```python
from build123d import *

# Parameters (mm, degrees)
F0_W          = 111
F0_H          = 107
F0_W_2        = 13
F0_H_2        = 5
F0_W_3        = 39
F0_H_3        = 7
F0_W_4        = 12
F0_H_4        = 1.5
F0_R          = 2.75
F0_W_5        = 4.5
F0_H_5        = 10
F0_H_6        = 15
F0_W_6        = 14
F0_W_7        = 17
F1_DEPTH      = 23
F2_W          = 111
F2_H          = 107
F3_DEPTH      = 3
F4_DEPTH      = 5
F5_DEPTH      = 13
F7_DEPTH      = 50
F9_DEPTH      = 10
F10_R         = 5
F11_T3_ANGLE  = 90
F11_T6_ANGLE  = 90
F11_T9_ANGLE  = 90
F11_T12_ANGLE = 90
F11_T15_DEPTH = 48
F11_T18_DEPTH = 48
F11_T21_DEPTH = 48
F11_T24_DEPTH = 48
F12_R         = 1


# Not quite as in the source:
# - a fillet or chamfer that OpenCascade refuses, or shapes differently, is made with other operations: its cross-section is extruded or revolved along the edge and cut away or added


with BuildPart() as f1:
    # F0 (on Top) → F1 (new body)
    with BuildSketch(Plane.XY):
        with Locations((55.5, 53.5)):
            Rectangle(F0_W, F0_H)
        with Locations((16.5, 12.5)):
            Rectangle(F0_W_2, F0_H_2, mode=Mode.SUBTRACT)
        Polygon((35.5980762114, 15), (36.4641016151, 13.5), (35.5980762114, 12), (33.8660254038, 12), (33, 13.5), (33.8660254038, 15), align=None, mode=Mode.SUBTRACT)
        with Locations((29.5, 28.5)):
            Rectangle(F0_W_3, F0_H_3, mode=Mode.SUBTRACT)
        with Locations((62.4641016151, 14.25)):
            Rectangle(F0_W_4, F0_H_4, mode=Mode.SUBTRACT)
        with Locations((71.75, 39.25)):
            Circle(F0_R, mode=Mode.SUBTRACT)
        with Locations((91.75, 37)):
            Rectangle(F0_W_5, F0_H_5, mode=Mode.SUBTRACT)
        with Locations((16.5, 59.5)):
            Rectangle(F0_W_2, F0_H_6, mode=Mode.SUBTRACT)
        with Locations((17, 89.5)):
            Rectangle(F0_W_6, F0_H_6, mode=Mode.SUBTRACT)
        with Locations((94.5, 59.5)):
            Rectangle(F0_W_2, F0_H_6, mode=Mode.SUBTRACT)
        with Locations((92.5, 93.5)):
            Rectangle(F0_W_7, F0_H_3, mode=Mode.SUBTRACT)
    extrude(amount=F1_DEPTH)

    # F2 (on face) → F3 (join)
    with BuildSketch(Plane(origin=(0, 0, 0), x_dir=(1, 0, 0), z_dir=(0, 0, -1))):
        with Locations((55.5, -53.5)):
            Rectangle(F2_W, F2_H)
    extrude(amount=-F3_DEPTH)

    # F4 (add): a face of the model
    f4_faces = [f1.faces().sort_by_distance(p)[0] for p in [
        (16.5, 12.5, 3),
    ]]
    extrude(f4_faces, amount=F4_DEPTH)

    # F5 (add): a face of the model
    f5_faces = [f1.faces().sort_by_distance(p)[0] for p in [
        (62.4641016151, 14.25, 3),
    ]]
    extrude(f5_faces, amount=F5_DEPTH)

    # F6 (on face) → F7 (join)
    with BuildSketch(Plane.YZ.offset(111)):
        with BuildLine():
            Line((11.0735931288, 23), (0, 23))
            Line((0, 23), (0, 0))
            Line((0, 0), (107, 0))
            Line((107, 0), (107, 23))
            Line((107, 23), (95.9264068712, 23))
            ThreePointArc((95.9264068712, 23), (53.5, 3), (11.0735931288, 23))
        make_face()
    extrude(amount=F7_DEPTH)

    # F8 (on face) → F9 (join)
    with BuildSketch(Plane.YZ.offset(161)):
        with BuildLine():
            Line((0, 23), (0, 0))
            Line((0, 0), (107, 0))
            Line((107, 0), (107, 23))
            Line((107, 23), (95.9264068712, 23))
            ThreePointArc((95.9264068712, 23), (53.5, 3), (11.0735931288, 23))
            Line((11.0735931288, 23), (0, 23))
        make_face()
        with BuildLine():
            Line((95.9264068712, 23), (11.0735931288, 23))
            ThreePointArc((11.0735931288, 23), (53.5, 3), (95.9264068712, 23))
        make_face()
    extrude(amount=F9_DEPTH)

    # F10
    f10_edges = [f1.edges().sort_by_distance(p)[0] for p in [
        (85.5, 107, 23),
        (171, 53.5, 23),
        (85.5, 0, 23),
        (0, 53.5, 23),
    ]]
    fillet(f10_edges, radius=F10_R)

    # F11: fillet of radius 10 on 4 edges, made by hand


with BuildPart() as f11_tool1:
    # F11_s2 → F11_t3 (revolve)
    with BuildSketch(Plane.YZ.offset(10)):
        with BuildLine():
            ThreePointArc((102, 23), (105.5355339059, 21.5355339059), (107, 18))
            Line((107, 18), (107, 23))
            Line((107, 23), (102, 23))
        make_face()
    revolve(axis=Axis((10, 97, 23), (0, 0, 1)), revolution_arc=F11_T3_ANGLE)


with BuildPart() as f11_tool4:
    # F11_s5 → F11_t6 (revolve)
    with BuildSketch(Plane.XZ.offset(-10)):
        with BuildLine():
            ThreePointArc((5, 23), (1.4644660941, 21.5355339059), (0, 18))
            Line((0, 18), (0, 23))
            Line((0, 23), (5, 23))
        make_face()
    revolve(axis=Axis((10, 10, 23), (0, 0, 1)), revolution_arc=F11_T6_ANGLE)


with BuildPart() as f11_tool7:
    # F11_s8 → F11_t9 (revolve)
    with BuildSketch(Plane.YZ.offset(161)):
        with BuildLine():
            ThreePointArc((5, 23), (1.4644660941, 21.5355339059), (0, 18))
            Line((0, 18), (0, 23))
            Line((0, 23), (5, 23))
        make_face()
    revolve(axis=Axis((161, 10, 23), (0, 0, 1)), revolution_arc=F11_T9_ANGLE)


with BuildPart() as f11_tool10:
    # F11_s11 → F11_t12 (revolve)
    with BuildSketch(Plane.XZ.offset(-97)):
        with BuildLine():
            ThreePointArc((166, 23), (169.5355339059, 21.5355339059), (171, 18))
            Line((171, 18), (171, 23))
            Line((171, 23), (166, 23))
        make_face()
    revolve(axis=Axis((161, 97, 23), (0, 0, 1)), revolution_arc=F11_T12_ANGLE)


with BuildPart() as f11_tool13:
    # F11_s14 → F11_t15 (new body)
    with BuildSketch(Plane.XY.offset(-25)):
        with BuildLine():
            ThreePointArc((161, 107), (168.0710678119, 104.0710678119), (171, 97))
            Line((171, 97), (171, 107))
            Line((171, 107), (161, 107))
        make_face()
    extrude(amount=F11_T15_DEPTH)


with BuildPart() as f11_tool16:
    # F11_s17 → F11_t18 (new body)
    with BuildSketch(Plane.XY.offset(23)):
        with BuildLine():
            ThreePointArc((161, 0), (168.0710678119, 2.9289321881), (171, 10))
            Line((171, 10), (171, 0))
            Line((171, 0), (161, 0))
        make_face()
    extrude(amount=-F11_T18_DEPTH)


with BuildPart() as f11_tool19:
    # F11_s20 → F11_t21 (new body)
    with BuildSketch(Plane.XY.offset(-25)):
        with BuildLine():
            ThreePointArc((0, 10), (2.9289321881, 2.9289321881), (10, 0))
            Line((10, 0), (0, 0))
            Line((0, 0), (0, 10))
        make_face()
    extrude(amount=F11_T21_DEPTH)


with BuildPart() as f11_tool22:
    # F11_s23 → F11_t24 (new body)
    with BuildSketch(Plane.XY.offset(23)):
        with BuildLine():
            ThreePointArc((0, 97), (2.9289321881, 104.0710678119), (10, 107))
            Line((10, 107), (0, 107))
            Line((0, 107), (0, 97))
        make_face()
    extrude(amount=-F11_T24_DEPTH)


with BuildPart() as f1_1:
    add(f1.part)

    # F11_t25: cut F11_tool1, F11_tool4, F11_tool7, F11_tool10, F11_tool13, F11_tool16, F11_tool19, F11_tool22
    add([f11_tool1.part, f11_tool4.part, f11_tool7.part, f11_tool10.part, f11_tool13.part, f11_tool16.part, f11_tool19.part, f11_tool22.part], mode=Mode.SUBTRACT)

    # F12
    f12_edges = [f1_1.edges().sort_by_distance(p)[0] for p in [
        (85.5, 102, 23),
        (164.535534, 100.535534, 23),
        (166, 53.5, 23),
        (164.535534, 6.464466, 23),
        (85.5, 5, 23),
        (6.464466, 6.464466, 23),
        (5, 53.5, 23),
        (6.464466, 100.535534, 23),
        (10, 12.5, 23),
        (16.5, 10, 23),
        (16.5, 15, 23),
        (23, 12.5, 23),
        (36.031089, 14.25, 23),
        (34.732051, 15, 23),
        (36.031089, 12.75, 23),
        (33.433013, 14.25, 23),
        (34.732051, 12, 23),
        (33.433013, 12.75, 23),
        (10, 28.5, 23),
        (29.5, 25, 23),
        (29.5, 32, 23),
        (49, 28.5, 23),
        (56.464102, 14.25, 23),
        (62.464102, 13.5, 23),
        (62.464102, 15, 23),
        (68.464102, 14.25, 23),
        (69, 39.25, 23),
        (89.5, 37, 23),
        (91.75, 32, 23),
        (91.75, 42, 23),
        (94, 37, 23),
        (136, 11.073593, 23),
        (111, 53.5, 23),
        (161, 53.5, 23),
        (136, 95.926407, 23),
        (10, 59.5, 23),
        (16.5, 52, 23),
        (16.5, 67, 23),
        (23, 59.5, 23),
        (17, 82, 23),
        (24, 89.5, 23),
        (10, 89.5, 23),
        (17, 97, 23),
        (94.5, 67, 23),
        (88, 59.5, 23),
        (101, 59.5, 23),
        (94.5, 52, 23),
        (92.5, 90, 23),
        (101, 93.5, 23),
        (84, 93.5, 23),
        (92.5, 97, 23),
    ]]
    fillet(f12_edges, radius=F12_R)


solid = f1_1.part
```
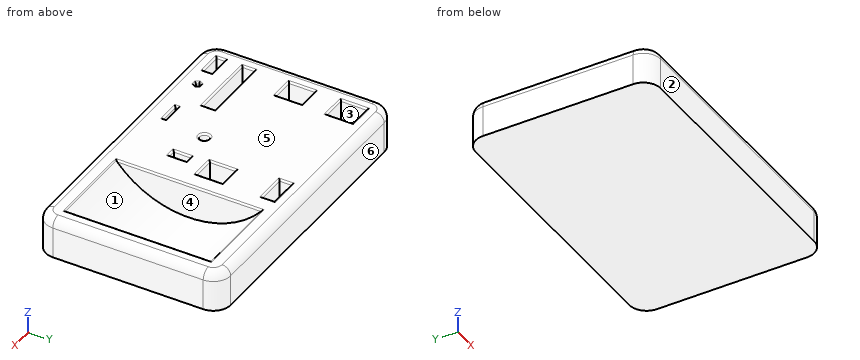
Geometry check sheet. Reference: the model listing, model coordinates, mm. Face numbers are marked on the shaded views. A direction names the side the tool comes from. Give positions to 0.01 mm unless a question says otherwise; leave off trailing zeros. Order: outer loops, then holes, each group sorted by start corner. A loop starts at its lowest first (then second) coordinate and runs counter-clockwise, first axis right, second up.
1. Gauge pin test, flat ends, axial feed: pin 1 Ø6.5 at (x, y) = (15.5, 63) entering from +Z; pin 2 Ø1 at (x, y) = (80, 58) entering from -Z; pin 3 Ø10.5 at (x, y) = (96.5, 61) entering from +Z. Record the tip position at first contact, or that the pin passes through.
2. Thickness scan on L1, parallel to X at y = 39.25, z = 10.75; L2, parallel to X at y = 66, z = 14.75; L3, parallel to X at y = 27, z = 15.25. Record the ranges inside material, lowest first.
3. Section check B-B, the plane y = 59. Enter the section's corners in (x, z).
4. Section check D-D, the plane z = 6. Give the number of separate pieces and of enclosed holes in the cut face, and give its area (3 significant figures).
5. Release check for a two-part mould opening along Y. For the marked faces 3, 4, 5 and 6 record: pulls with the +Y half, pulls with the -Y half, needs draft (parallel to the pull), parting line crosses it, or undercut.
6. Access from +Z, -Z, +X, -X, +Y, -Y to the whole of each face (thin tool, end or side, straight path). Record for the marked faces 1 and 2.
7. Section check A-A, the plane x = 156. Enter the section's corners in (y, z).
Values follow:
1. pin 1: stops at z = 3
1. pin 2: stops at z = 0
1. pin 3: stops at z = 22.97
2. L1: x = 0 to 69, 74.5 to 89.5, 94 to 111, 161 to 171
2. L2: x = 0 to 10, 23 to 88, 101 to 111, 161 to 171
2. L3: x = 0 to 10, 49 to 111, 161 to 171
3. outline: (0, 0) - (171, 0) - (171, 18) arc R5 ccw to (166, 23) - (162, 23) arc R1 ccw to (161, 22) - (161, 3.28) - (111, 3.28) - (111, 22) arc R1 ccw to (110, 23) - (102, 23) arc R1 ccw to (101, 22) - (101, 3) - (88, 3) - (88, 22) arc R1 ccw to (87, 23) - (24, 23) arc R1 ccw to (23, 22) - (23, 3) - (10, 3) - (10, 22) arc R1 ccw to (9, 23) - (5, 23) arc R5 ccw to (0, 18) - close
4. separate pieces: 1
4. enclosed holes: 9
4. area: 15,400 mm2
5. face 3: undercut
5. face 4: undercut
5. face 5: needs draft
5. face 6: pulls with the +Y half
6. face 1: +Z
6. face 2: +Z, -Z, +X, -X, -Y
7. outline: (0, 0) - (107, 0) - (107, 18) arc R5 ccw to (102, 23) - (96.4, 23) arc R1 ccw to (95.63, 22.64) arc R55 cw to (11.37, 22.64) arc R1 ccw to (10.6, 23) - (5, 23) arc R5 ccw to (0, 18) - close
